Design review of the part built by this model. Coordinates are the model's own, in mm. A direction names the side the tool comes from. Coordinates: 2 decimals unless noted, no trailing zeros. Loops run counter-clockwise (first coordinate to the right, second up) from the corner with the lowest first, then second, coordinate; pieces in that order, holes last. Notation, with made-up numbers: (80.25, 0.5) - (95.25, 0.5) arc R22 ccw to (95.25, 30.5) - close; hole circle Ø9 at (14.25, 81). An arc over 180 degrees is marked (long way). Answer in a Markdown table with one row per item. Add a question column.
(1) To check wall thickness, follow L1, parallel to X at y = 2.95, z = 0; L2, parallel to Y at x = -10.25, z = 0; L3, parallel to Y at x = -8, z = 0. State the ranges of each line that lie inside material, in increasing order. Write a range as [from, to].
(2) The part is to be moulded in two halves that separate along Z. For faces 1 (the face through (-9.208, 290.307, -4.436)), 2 (the face through (-6, 282, 0)), 3 (the face through (0, 6, -9)), say which applies: released by +Z, released by -Z, zero draft, split by the parting line, or undercut.
(3) Clearance check with flat-ended pins moving along their axes: pin 1 (1 mm diameter, centred on x = -3.5, y = 105.5, fed in from -Z); pin 2 (1.5 mm diameter, centred on y = 124, z = -4.5, fed in from +X); pin 3 (9 mm diameter, centred on y = 288, z = 0, fed in from +X); pin 4 (6.5 mm diameter, centred on x = 1.5, y = 15, fed in from +Z). State where each tip first meets the part, or that it passes through.
(4) We need section A-A, the plane y = 288. Write out the cut boundary in (x, z).
(5) We need section B-B, the plane x = 0. Write out the cut boundary in (y, z).
(6) We need section C-C, the plane y = 48. Write out the cut boundary in (x, z), plus the area to 3 significant figures.
(7) For faces 4 (the face through (0, 8, -3)), 5 (the face through (4, 34, 5)), 6 (the face through (6, 282, 0)), 7 (the face through (0, 2, -6)), list the 3-axis set-ups (+Z, -Z, +X, -X, +Y, -Y) from which the entire face can be reached by the end or side of a thin tool; tool diameter is ignored.
from build123d import *

# Parameters (mm, degrees)
F0_R           = 12.5
F1_DEPTH       = 300
F2_W           = 12
F2_H           = 50
F3_DEPTH       = 12.501
F3_DEPTH_BACK  = 12.501
F4_R           = 5
F5_DEPTH       = 12.501
F5_DEPTH_BACK  = 12.501
F7_DEPTH       = 4
F7_DEPTH_BACK  = 4
F10_DEPTH      = 2
F10_DEPTH_BACK = 2
F11_R          = 6
F12_DEPTH      = 8
F13_R          = 1.5
F15_SIZE       = 1
F18_R          = 1
F19_DEPTH      = 17.076317684


with BuildPart() as f1:
    # F0 (on Front) → F1 (new body)
    with BuildSketch(Plane.XZ):
        Circle(F0_R)
    extrude(amount=-F1_DEPTH)

    # F2 (on Top) → F3 (cut, two sides)
    with BuildSketch(Plane.XY) as f3_sk:
        with Locations((0, 300)):
            Rectangle(F2_W, F2_H)
    extrude(amount=-F3_DEPTH, mode=Mode.SUBTRACT)
    extrude(f3_sk.sketch, amount=F3_DEPTH_BACK, mode=Mode.SUBTRACT)

    # F4 (on Right) → F5 (cut, two sides)
    with BuildSketch(Plane.YZ) as f5_sk:
        with Locations((288, 0)):
            Circle(F4_R)
    extrude(amount=-F5_DEPTH, mode=Mode.SUBTRACT)
    extrude(f5_sk.sketch, amount=F5_DEPTH_BACK, mode=Mode.SUBTRACT)

    # F6 (on Right) → F7 (cut, two sides)
    with BuildSketch(Plane.YZ) as f7_sk:
        with BuildLine():
            Line((0, 43.2144903421), (0, -2))
            Line((0, -2), (35, -2))
            ThreePointArc((35, -2), (56.2132034356, 6.7867965644), (65, 28))
            Line((65, 28), (65, 43.2144903421))
            Line((65, 43.2144903421), (0, 43.2144903421))
        make_face()
    extrude(amount=F7_DEPTH, mode=Mode.SUBTRACT)
    extrude(f7_sk.sketch, amount=-F7_DEPTH_BACK, mode=Mode.SUBTRACT)

    # F9 (on offset) → F10 (cut, two sides)
    with BuildSketch(Plane.XZ.offset(-6)) as f10_sk:
        with BuildLine():
            Line((-9, 23.9692713934), (-9, 0))
            ThreePointArc((-9, 0), (0, -9), (9, 0))
            Line((9, 0), (9, 23.9692713934))
            Line((9, 23.9692713934), (-9, 23.9692713934))
        make_face()
    extrude(amount=-F10_DEPTH, mode=Mode.SUBTRACT)
    extrude(f10_sk.sketch, amount=F10_DEPTH_BACK, mode=Mode.SUBTRACT)

    # F11 (on Front) → F12 (cut, through all)
    with BuildSketch(Plane.XZ):
        Circle(F11_R)
    extrude(amount=-F12_DEPTH, mode=Mode.SUBTRACT)

    # F13 (on Top) → F14 (revolve, cut)
    with BuildSketch(Plane.XY):
        with Locations((12.5, 6)):
            Circle(F13_R)
    revolve(axis=Axis((0, 7.8222351149, 0), (0, 1, 0)), mode=Mode.SUBTRACT)

    # F15
    f15_edges = [f1.edges().sort_by_distance(p)[0] for p in [
        (0, 0, -12.5),
    ]]
    chamfer(f15_edges, length=F15_SIZE)

    # F18 (on line) → F19 (cut, through all)
    with BuildSketch(Plane(origin=(0, 0, 0), x_dir=(0, -1, 0), z_dir=(-0.8660254038, 0, 0.5))):
        with Locations((-6, 0)):
            Circle(F18_R)
    extrude(amount=F19_DEPTH, mode=Mode.SUBTRACT)


solid = f1.part
Responses:
| question | item | result |
|---|---|---|
| 1 | L1 | x = [-12.5, -6], [6, 12.5] |
| 1 | L2 | y = [0, 283], [293, 300] |
| 1 | L3 | y = [0, 4], [8, 283], [293, 300] |
| 2 | face 1 | undercut |
| 2 | face 2 | zero draft |
| 2 | face 3 | released by +Z |
| 3 | pin 1 | stops at z = -12.13 |
| 3 | pin 2 | stops at x = 11.92 |
| 3 | pin 3 | passes through |
| 3 | pin 4 | stops at z = 11.84 |
| 4 | outline | (-11.46, -5) arc R12.5 ccw to (-6, -10.97) - (-6, -5) - close; (-11.46, 5) - (-6, 5) - (-6, 10.97) arc R12.5 ccw to start; (6, -10.97) arc R12.5 ccw to (11.46, -5) - (6, -5) - close; (6, 5) - (11.46, 5) arc R12.5 ccw to (6, 10.97) - close |
| 5 | outline | (0, -11.5) - (1, -12.5) - (4.5, -12.5) arc R1.5 cw to (7.5, -12.5) - (275, -12.5) - (275, 12.5) - (60.69, 12.5) arc R30 cw to (35, -2) - (8, -2) - (8, -9) - (4, -9) - (4, -6) - (0, -6) - close |
| 6 | outline | (-4, 0.96) - (-4, 11.84) arc R12.5 ccw (long way) to (4, 11.84) - (4, 0.96) - close |
| 6 | area | 400 mm2 |
| 7 | face 4 | +Z |
| 7 | face 5 | +Z, -Y |
| 7 | face 6 | +Z, -Z, +Y |
| 7 | face 7 | -Y |
